Build history of the part. All positions in model axes, mm. Face numbers are marked on the shaded views. Give positions to 0.01 mm unless a question says otherwise; leave off trailing zeros. Write each loop counter-clockwise with the first axis right and the second up, starting at its lowest first coordinate (ties: lowest second). Pieces come first, ordered by that corner, then holes. Notation, with made-up numbers: (-27.75, 59.25) -> (2.25, 59.25) arc R17 cw to (2.25, 67.25) -> close; hole circle Ø10 at (7, 73.25). An arc over 180 degrees is marked (long way). Write item = value, one per line. Start each with the question number.
Q1. Mould opens along X. For the marked faces 1, 2, 3 and 4 say: pulls with the +X half, pulls with the -X half, needs draft (parallel to the pull), parting line crosses it, or undercut.
Q2. Saw through at A-A, the plane y = 26.5. List the corners of the cut face in (x, z), then the cut area to 3 significant figures.
Q3. Saw through at B-B, the plane x = 0. List the corners of the cut face in (y, z), then the cut area to 3 significant figures.
Q4. Wall check: line 1 (Y direction, x = 3.5, z = -26); line 2 (Z direction, x = -1, y = 2); line 3 (Z direction, x = -3, y = 17). Give the ranges that are in metal, low to high.
from build123d import *

# Parameters (mm, degrees)
SKETCH1_W           = 44.8
SKETCH1_H           = 59.4
BOSS_EXTRUDE1_DEPTH = 30
CUT_EXTRUDE1_DEPTH  = 27
CUT_EXTRUDE2_DEPTH  = 46.965748117


with BuildPart() as part:
    # Sketch1 → Boss-Extrude1 (new body)
    with BuildSketch(Plane(origin=(0, 0, 0), x_dir=(1, 0, 0), z_dir=(0, 1, 0))):
        Rectangle(SKETCH1_W, SKETCH1_H)
    extrude(amount=BOSS_EXTRUDE1_DEPTH)

    # Sketch3 → Cut-Extrude1 (cut)
    with BuildSketch(Plane(origin=(0, 30, 0), x_dir=(1, 0, 0), z_dir=(0, 1, 0))):
        with BuildLine():
            Line((-4.5, 23.8), (-4.5, 30.7))
            Line((-4.5, 30.7), (4.5, 30.7))
            Line((4.5, 30.7), (4.5, 23.8))
            ThreePointArc((4.5, 23.8), (0, 19.3), (-4.5, 23.8))
        make_face()
        with BuildLine():
            Line((-4.5, -23.8), (-4.5, -30.7))
            Line((-4.5, -30.7), (4.5, -30.7))
            Line((4.5, -30.7), (4.5, -23.8))
            ThreePointArc((4.5, -23.8), (0, -19.3), (-4.5, -23.8))
        make_face()
    extrude(amount=-CUT_EXTRUDE1_DEPTH, mode=Mode.SUBTRACT)

    # Sketch4 → Cut-Extrude2 (cut, through all)
    with BuildSketch(Plane(origin=(0, 3, 0), x_dir=(1, 0, 0), z_dir=(0, 1, 0))):
        with BuildLine():
            Line((-2.35, 23.8), (-2.35, 29.7))
            Line((-2.35, 29.7), (2.35, 29.7))
            Line((2.35, 29.7), (2.35, 23.8))
            ThreePointArc((2.35, 23.8), (0, 21.45), (-2.35, 23.8))
        make_face()
        with BuildLine():
            Line((-2.35, -23.8), (-2.35, -29.7))
            Line((-2.35, -29.7), (2.35, -29.7))
            Line((2.35, -29.7), (2.35, -23.8))
            ThreePointArc((2.35, -23.8), (0, -21.45), (-2.35, -23.8))
        make_face()
    extrude(amount=-CUT_EXTRUDE2_DEPTH, mode=Mode.SUBTRACT)


solid = part.part
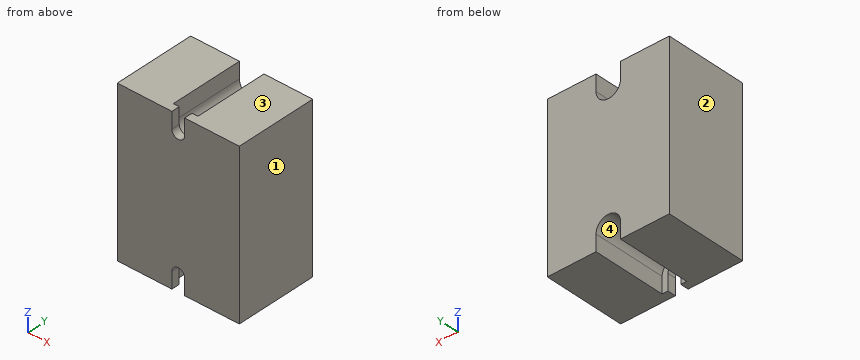
Report:
q1.face_1 = pulls with the +X half
q1.face_2 = pulls with the -X half
q1.face_3 = needs draft
q1.face_4 = undercut
q2.outline = (-22.4, -29.7) -> (-4.5, -29.7) -> (-4.5, -23.8) arc R4.5 cw to (4.5, -23.8) -> (4.5, -29.7) -> (22.4, -29.7) -> (22.4, 29.7) -> (4.5, 29.7) -> (4.5, 23.8) arc R4.5 cw to (-4.5, 23.8) -> (-4.5, 29.7) -> (-22.4, 29.7) -> close
q2.area = 2,490 mm2
q3.outline = (0, -21.45) -> (3, -21.45) -> (3, -19.3) -> (30, -19.3) -> (30, 19.3) -> (3, 19.3) -> (3, 21.45) -> (0, 21.45) -> close
q3.area = 1,170 mm2
q4.line_1 = 0 to 3
q4.line_2 = -21.67 to 21.67
q4.line_3 = -20.45 to 20.45
